Autodesk Inventor part; units mm, degrees
sketch "Эскиз1" plane through (0, 0, 0) normal (0, 0, 1) x (1, 0, 0)
  arc A0 (-20, -20) -> (-10, -30) centre (-10, -20) ccw
  line L0 (-20, 20) -> (-20, -20)
  arc A1 (-10, 30) -> (-20, 20) centre (-10, 20) ccw
  line L1 (10, 30) -> (-10, 30)
  arc A2 (20, 20) -> (10, 30) centre (10, 20) ccw
  line L2 (20, -20) -> (20, 20)
  arc A3 (10, -30) -> (20, -20) centre (10, -20) ccw
  line L3 (-10, -30) -> (10, -30)
  arc A4 (10, -35) -> (25, -20) centre (10, -20) ccw
  line L4 (25, -20) -> (25, 20)
  arc A5 (25, 20) -> (10, 35) centre (10, 20) ccw
  line L5 (10, 35) -> (-10, 35)
  arc A6 (-10, 35) -> (-25, 20) centre (-10, 20) ccw
  line L6 (-25, 20) -> (-25, -20)
  arc A7 (-25, -20) -> (-10, -35) centre (-10, -20) ccw
  line L7 (-10, -35) -> (10, -35)
  dimension "d4" = 5
extrude "Выдавливание1" add sketch "Эскиз1" along normal mid plane 30
properties part number "Козырёк_версия_2"
CAD build for the part. Positions are in the model's coordinates, mm. A direction names the side the tool comes from. Coordinates: 2 decimals unless noted, no trailing zeros. Loops run counter-clockwise (first coordinate to the right, second up) from the corner with the lowest first, then second, coordinate; pieces in that order, holes last. Notation, with made-up numbers: (31.5, 39) - (65.5, 39) arc R28 cw to (65.5, 58) - close; hole circle Ø7 at (32, -10.75). An arc over 180 degrees is marked (long way). Use one line per item in the form item = value. Start each with the question number.
1) Band-saw the part on B-B (x = 5). Give the cut face in (y, z).
2) Band-saw the part on C-C (z = 4.75). Give the cut face in (x, y), and give its area (3 significant figures).
3) Tool access for faces 1 (the face through (-20.49, -30.72, -0.21)), 2 (the face through (0, -30, 0)): list every direction of +Z, -Z, +X, -X, +Y, -Y with a clear straight run to the whole face (end or side of a thin tool).
4) Drill centre lines: L1, parallel to Y at x = 1.5, z = -3.5; L2, parallel to X at y = -9.5, z = 11.5; L3, parallel to Y at x = -11, z = 4.75. Where is each one in solid material? Low to high. Write a range as from..to.
5) Flat gauge pins, fed straight in: pin 1 (1.5 mm diameter, centred on y = -28, z = -8, fed in from +X); pin 2 (2 mm diameter, centred on x = -19, z = 0.5, fed in from +Y); pin 3 (1 mm diameter, centred on x = 18, z = 4, fed in from +Y). Where does each tip first touch, or does it go through?
6) Band-saw the part on A-A (y = -1.5). Give the cut face in (x, z), and give its area (3 significant figures).
7) Two-plate mould, pull along Y, no slides. Class faces 3 (the face through (20.49, 30.72, -0.21)), 4 (the face through (0, 30, 0)), 5 (the face through (-25, 0, 0)): +Y half, -Y half, draft (parallel to the pull), parting line (faces both ways), or undercut.
Check values:
q1.outline = (-35, -15) - (-30, -15) - (-30, 15) - (-35, 15) - close; (30, -15) - (35, -15) - (35, 15) - (30, 15) - close
q2.outline = (-25, -20) arc R15 ccw to (-10, -35) - (10, -35) arc R15 ccw to (25, -20) - (25, 20) arc R15 ccw to (10, 35) - (-10, 35) arc R15 ccw to (-25, 20) - close; hole (-20, -20) arc R10 ccw to (-10, -30) - (10, -30) arc R10 ccw to (20, -20) - (20, 20) arc R10 ccw to (10, 30) - (-10, 30) arc R10 ccw to (-20, 20) - close
q2.area = 993 mm2
q3.face_1 = +Z, -Z, -X, -Y
q3.face_2 = +Z, -Z
q4.L1 = -35..-30, 30..35
q4.L2 = -25..-20, 20..25
q4.L3 = -34.97..-29.95, 29.95..34.97
q5.pin_1 = 23.13
q5.pin_2 = 32.69
q5.pin_3 = 32.99
q6.outline = (-25, -15) - (-20, -15) - (-20, 15) - (-25, 15) - close; (20, -15) - (25, -15) - (25, 15) - (20, 15) - close
q6.area = 300 mm2
q7.face_3 = +Y half
q7.face_4 = undercut
q7.face_5 = draft
